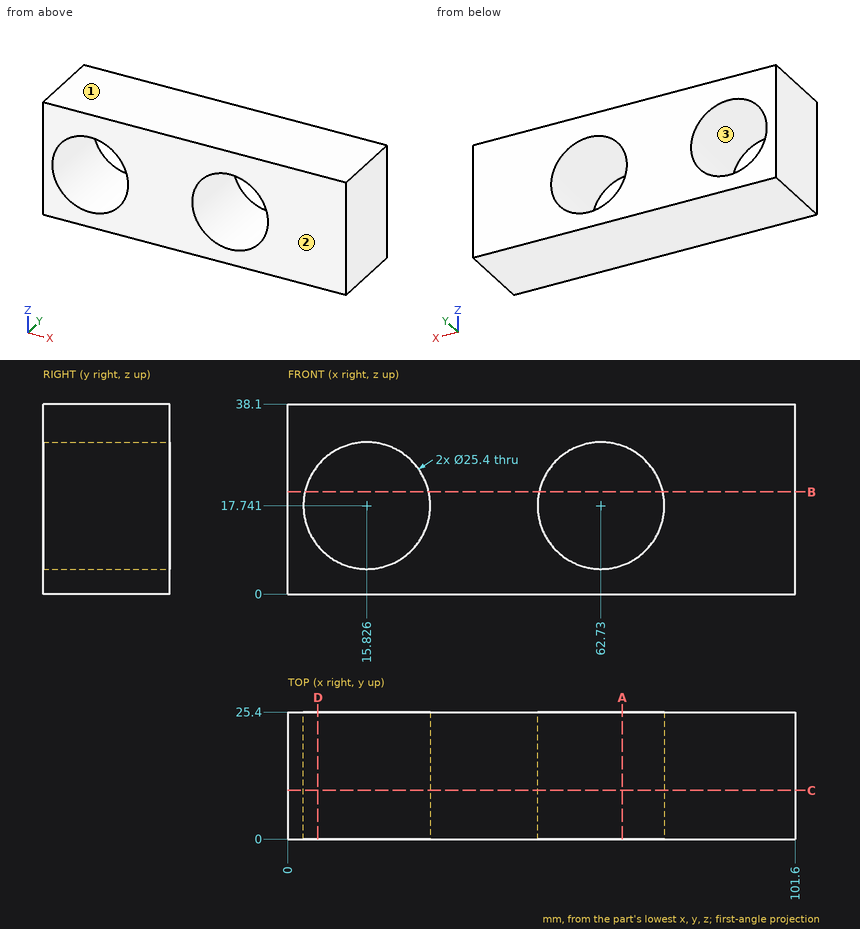
Drawing for the job (mm, zero at the part's lowest x, y, z). Give positions to 0.01 mm unless a question says otherwise; leave off trailing zeros. Order: outer loops, then holes, each group sorted by start corner. A loop starts at its lowest first (then second) coordinate and runs counter-clockwise, first axis right, second up. Notation, with made-up numbers: (-25.75, 65) - (0.25, 65) arc R9 cw to (0.25, 72) - close; hole circle Ø8 at (47.25, -21). An arc over 180 degrees is marked (long way). Write item = value, one per line. Start each with the question number.
1. Cut at B-B, the plane z = 20.5. List the corners of the cut face in (x, y), and give its area (3 significant figures).
2. Cut at A-A, the plane x = 67. List the corners of the cut face in (y, z), and give its area (3 significant figures).
3. Cut at C-C, the plane y = 9.75. List the corners of the cut face in (x, z), and give its area (3 significant figures).
4. Cut at D-D, the plane x = 6. List the corners of the cut face in (y, z) (1 decimal).
5. Two-plate mould, pull along Z, no slides. Class the marked faces 1, 2 and 3: pulls with the +Z half, pulls with the -Z half, needs draft (parallel to the pull), parting line crosses it, or undercut.
6. Probe line 1 along X through (y, z) = (20.5, 29.5) (1 decimal); line 2 along X through (y, z) = (21.5, 22) (1 decimal); line 3 along Z through (x, y) = (27, 4.75) (1 decimal). List the from-to ranges inside material, lowest first.
7. Drop a flat-ended pin along its axis: P1, Ø2, axis at y = 13, z = 31.5, coming from the -X side. Give the stop position or say it passes through.
Taken from the geometry:
q1.outline = (0, 0) - (3.43, 0) - (3.43, 25.4) - (0, 25.4) - close; (28.22, 0) - (50.33, 0) - (50.33, 25.4) - (28.22, 25.4) - close; (75.13, 0) - (101.6, 0) - (101.6, 25.4) - (75.13, 25.4) - close
q1.area = 1,320 mm²
q2.outline = (0, 0) - (25.4, 0) - (25.4, 5.78) - (0, 5.78) - close; (0, 29.7) - (25.4, 29.7) - (25.4, 38.1) - (0, 38.1) - close
q2.area = 360 mm²
q3.outline = (0, 0) - (101.6, 0) - (101.6, 38.1) - (0, 38.1) - close; hole circle Ø25.4 at (15.83, 17.74); hole circle Ø25.4 at (62.73, 17.74)
q3.area = 2,860 mm²
q4.outline = (0, 0) - (25.4, 0) - (25.4, 9.7) - (0, 9.7) - close; (0, 25.8) - (25.4, 25.8) - (25.4, 38.1) - (0, 38.1) - close
q5.face_1 = pulls with the +Z half
q5.face_2 = needs draft
q5.face_3 = undercut
q6.line_1 = 0 to 11, 20.6 to 57.9, 67.5 to 101.6
q6.line_2 = 0 to 3.9, 27.8 to 50.8, 74.7 to 101.6
q6.line_3 = 0 to 11.7, 23.8 to 38.1
q7.P1 = 0
